The drawing under review shows one solid part. Ordinate dimensions are in mm from its lowest x, y, z. Round coordinates to 2 decimals unless told otherwise and drop trailing zeros. Loops run counter-clockwise (first coordinate to the right, second up) from the corner with the lowest first, then second, coordinate; pieces in that order, holes last. Notation, with made-up numbers: M 27,54.5 L 40,54.5 A26 cw 40,90.5 Z; hole C 88,-2.5 d9. An arc over 180 degrees is marked long. Use a Markdown table: item, result.
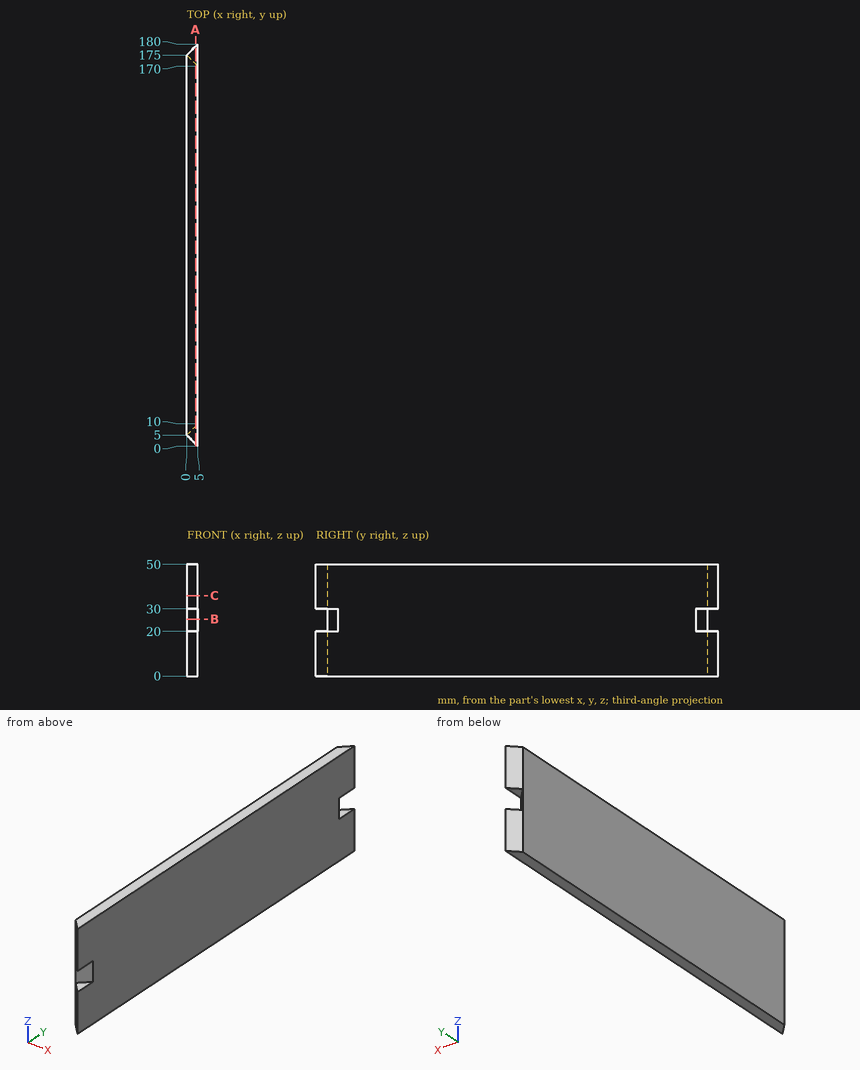
1. Take a section at C-C on z = 36. Give the boundary of the cut face in (x, y).
Check values:
| item | result |
|---|---|
| outline | M 0,5 L 5,0 L 5,180 L 0,175 Z |
2. Take a section at B-B on z = 25.5. Give the boundary of the cut face in (x, y), and give its area (3 significant figures).
Check values:
| item | result |
|---|---|
| outline | M 0,5 L 5,10 L 5,170 L 0,175 Z |
| area | 825 mm² |
3. Wall thickness on line 1 along Y through (x, z) = (3.75, 32.5); line 2 along Y through (x, z) = (0.95, 9): over which ranges is each line inside the solid? List them lowest first. Write a range as from..to.
Check values:
| item | result |
|---|---|
| line 1 | y = 1.25..178.75 |
| line 2 | y = 4.05..175.95 |
4. Take a section at A-A on x = 3.95. Give the boundary of the cut face in (y, z), and give its area (3 significant figures).
Check values:
| item | result |
|---|---|
| outline | M 1.05,0 L 178.95,0 L 178.95,20 L 171.05,20 L 171.05,30 L 178.95,30 L 178.95,50 L 1.05,50 L 1.05,30 L 8.95,30 L 8.95,20 L 1.05,20 Z |
| area | 8,740 mm² |
5. Insertion check: pin 1 (2 mm diameter, centred on x = 2.5, z = 32, fed in from +Y). The pin has a flat end and moves straight along its axis. Give the tip position at first contact, or say it passes through.
Check values:
| item | result |
|---|---|
| pin 1 | stops at y = 178.5 |
